from build123d import *

# Parameters (mm, degrees)
F0_W     = 38
F0_H     = 53.5
F1_DEPTH = 13.5
F2_W     = 35
F2_H     = 50.5
F3_DEPTH = 12.5
F4_R     = 2
F5_DEPTH = 25
F6_W     = 9
F6_H     = 6.5
F7_DEPTH = 25
F8_W     = 10
F8_H     = 5
F9_DEPTH = 2


with BuildPart() as f1:
    # F0 (on Top) → F1 (new body)
    with BuildSketch(Plane.XY):
        Rectangle(F0_W, F0_H)
    extrude(amount=F1_DEPTH)

    # F2 (on face) → F3 (cut)
    with BuildSketch(Plane.XY.offset(13.5)):
        Rectangle(F2_W, F2_H)
    extrude(amount=-F3_DEPTH, mode=Mode.SUBTRACT)

    # F4 (on face) → F5 (cut)
    with BuildSketch(Plane(origin=(0, 0, 0), x_dir=(1, 0, 0), z_dir=(0, 0, -1))):
        with Locations((-4, -14.75)):
            Circle(F4_R)
    extrude(amount=-F5_DEPTH, mode=Mode.SUBTRACT)

    # F6 (on face) → F7 (cut)
    with BuildSketch(Plane.XZ.offset(26.75)):
        with Locations((-7, 10.25)):
            Rectangle(F6_W, F6_H)
    extrude(amount=-F7_DEPTH, mode=Mode.SUBTRACT)

    # F8 (on face) → F9 (join)
    with BuildSketch(Plane.XY.offset(1)):
        with Locations((0, 2.75)):
            Rectangle(F8_W, F8_H)
    extrude(amount=F9_DEPTH)


solid = f1.part
Check sheet for the modelled part. Datum: model origin and axes. Units: mm. A direction names the side the tool comes from. Round coordinates to 2 decimals unless told otherwise and drop trailing zeros. Loops run counter-clockwise (first coordinate to the right, second up) from the corner with the lowest first, then second, coordinate; pieces in that order, holes last. Notation, with made-up numbers: (-38.5, -29) - (-18.5, -29) arc R33 cw to (-18.5, 7) - close; hole circle Ø6 at (39.5, 28). An arc over 180 degrees is marked (long way). Answer as CSV lines item,"result". Start each with the question number.
Item 1: Scan lines: line 1 (X direction, y = -9, z = 10.5); line 2 (Y direction, x = 8, z = 9.5); line 3 (Y direction, x = -4, z = 0.5). Record each from-to range of solid material in increasing order. Write a range as [from, to].
Item 2: Section check D-D (y = 14.75). Record the boundary of the cut face in (x, z), and give its area (3 significant figures).
Item 3: Release check for a two-part mould opening along X. For faces 1 (the flat face through (-2.5, -26, 10)), 2 (the flat face through (0, 26.75, 7)), 3 (the flat face through (19, 0, 7)) record: +X half, -X half, draft (parallel to the pull), parting line (faces both ways), or undercut.
Item 4: Depth check by flat-ended pin: P1, Ø5.5, axis at x = 1.5, y = 2.5, coming from the +Z side; P2, Ø0.8, axis at x = -7.5, y = -26.5, coming from the +Z side; P3, Ø10.5, axis at x = -7.5, y = -7.5, coming from the +Z side. Enter the tip coordinate at first touch or a pass-through.
Item 5: Section check C-C (z = 5.5). Record the boundary of the cut face in (x, y).
Item 6: Section check A-A (z = 1.75). Record the boundary of the cut face in (x, y), and give its area (4 significant figures).
Item 7: Section check B-B (x = -4). Record the boundary of the cut face in (y, z), and give its area (4 significant figures).
Item 8: Set-up check for faces 4 (the flat face through (0, 5.25, 2)), 5 (the flat face through (-11.5, -26, 10)), 6 (the cylindrical face through (-4.26, 12.767, 0.493)): record each of +Z, -Z, +X, -X, +Y, -Y from which the full face is reachable in a straight line by a thin tool's end or side.
Report:
1,line 1,"x = [-19, -17.5], [17.5, 19]"
1,line 2,"y = [-26.75, -25.25], [25.25, 26.75]"
1,line 3,"y = [-26.75, 12.75], [16.75, 26.75]"
2,outline,"(-19, 0) - (-6, 0) - (-6, 1) - (-17.5, 1) - (-17.5, 13.5) - (-19, 13.5) - close; (-2, 0) - (19, 0) - (19, 13.5) - (17.5, 13.5) - (17.5, 1) - (-2, 1) - close"
2,area,"71.5 mm2"
3,face 1,"undercut"
3,face 2,"draft"
3,face 3,"+X half"
4,P1,"stops at z = 3"
4,P2,"stops at z = 7"
4,P3,"stops at z = 1"
5,outline,"(-19, -26.75) - (19, -26.75) - (19, 26.75) - (-19, 26.75) - close; hole (-17.5, -25.25) - (17.5, -25.25) - (17.5, 25.25) - (-17.5, 25.25) - close"
6,outline,"(-19, -26.75) - (19, -26.75) - (19, 26.75) - (-19, 26.75) - close; (-5, 0.25) - (5, 0.25) - (5, 5.25) - (-5, 5.25) - close; hole (-17.5, -25.25) - (17.5, -25.25) - (17.5, 25.25) - (-17.5, 25.25) - close"
6,area,"315.5 mm2"
7,outline,"(-26.75, 0) - (12.75, 0) - (12.75, 1) - (5.25, 1) - (5.25, 3) - (0.25, 3) - (0.25, 1) - (-25.25, 1) - (-25.25, 7) - (-26.75, 7) - close; (16.75, 0) - (26.75, 0) - (26.75, 13.5) - (25.25, 13.5) - (25.25, 1) - (16.75, 1) - close"
7,area,"87.25 mm2"
8,face 4,"+Z"
8,face 5,"+Z, -Y"
8,face 6,"+Z, -Z"
